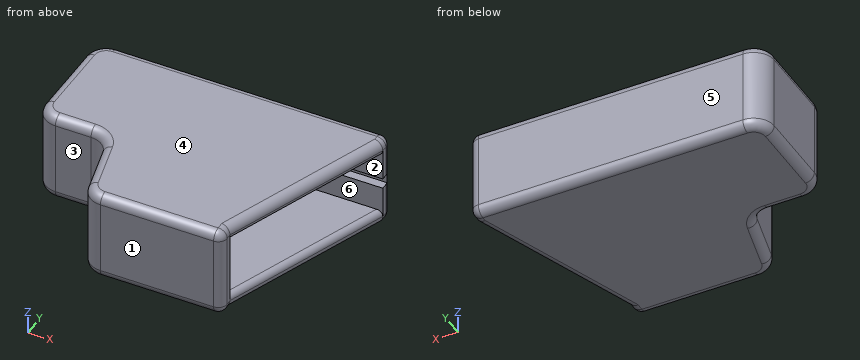
from build123d import *

# Parameters (mm, degrees)
F1_DEPTH = 21
F4_DEPTH = 5
F5_DEPTH = 5
F6_R     = 7
F7_R     = 3
F9_DEPTH = 3
F10_R    = 1.99999


# Not quite as in the source:
# - a fillet or chamfer is up to 0.001 mm smaller than in the source, because OpenCascade refuses the exact size


with BuildPart() as f1:
    # F0 (on Top) → F1 (new body)
    with BuildSketch(Plane.XY):
        Polygon((-23.5, 30), (71.5, 30), (71.5, 35), (-28.5, 35), (-28.5, -5), (-3.906596233, -5), (3.1079638678, -33.1388689644), (50.2020280941, -33.1388689644), (50.0145601007, -28.1388689644), (7.0145601007, -28.1388689644), (0, 0), (-23.5, 0), align=None)
    extrude(amount=F1_DEPTH)

    # F3 (on face) → F4 (join)
    with BuildSketch(Plane.XY.offset(21)):
        Polygon((71.5, 35), (-28.5, 35), (-28.5, -5), (-3.906596233, -5), (3.1079638678, -33.1388689644), (50.2020280941, -33.1388689644), (50.0145601007, -28.1388689644), (71.5, 30), align=None)
    extrude(amount=F4_DEPTH)

    # F2 (on face) → F5 (join)
    with BuildSketch(Plane(origin=(0, 0, 0), x_dir=(1, 0, 0), z_dir=(0, 0, -1))):
        Polygon((-28.5, -35), (71.5, -35), (71.5, -30), (50.0145601007, 28.1388689644), (50.2020280941, 33.1388689644), (3.1079638678, 33.1388689644), (-3.906596233, 5), (-28.5, 5), align=None)
    extrude(amount=F5_DEPTH)

    # F6
    f6_edges = [f1.edges().sort_by_distance(p)[0] for p in [
        (0, 0, 10.5),
        (-3.906596, -5, 10.5),
        (7.01456, -28.138869, 10.5),
        (3.107964, -33.138869, 10.5),
        (-28.5, -5, 10.5),
        (-28.5, 35, 10.5),
        (-23.5, 0, 10.5),
    ]]
    fillet(f6_edges, radius=F6_R)

    # F7
    f7_edges = [f1.edges().sort_by_distance(p)[0] for p in [
        (25, 35, 26),
        (25, 35, -5),
        (71.5, 35, 10.5),
        (-26.449747, 32.949747, 26),
        (71.5, 32.5, 26),
        (-28.5, 15, 26),
        (60.75728, 0.930566, 26),
        (-26.449747, -2.949747, 26),
        (50.108294, -30.638869, 26),
        (-15.437915, -5, 26),
        (29.389613, -33.138869, 26),
        (-5.066085, -6.484015, 26),
        (4.267453, -31.654854, 26),
        (-0.399316, -19.069434, 26),
        (-15.437915, -5, -5),
        (-5.066085, -6.484015, -5),
        (-26.449747, -2.949747, -5),
        (-0.399316, -19.069434, -5),
        (-28.5, 15, -5),
        (4.267453, -31.654854, -5),
        (-26.449747, 32.949747, -5),
        (29.389613, -33.138869, -5),
        (50.108294, -30.638869, -5),
        (71.5, 32.5, -5),
        (60.75728, 0.930566, -5),
        (50.202028, -33.138869, 10.5),
    ]]
    fillet(f7_edges, radius=F7_R)

    # F8 (on face) → F9 (cut)
    with BuildSketch(Plane.XZ.offset(-30)):
        Polygon((-23.5, 12.25), (-23.5, 10.5), (-23.5, 8.75), (74.1642639041, 8.75), (74.1642639041, 12.25), align=None)
    extrude(amount=-F9_DEPTH, mode=Mode.SUBTRACT)

    # F10 (radius 2 in the source; OpenCascade refuses exactly that, so slightly less here)
    f10_edges = [f1.edges().sort_by_distance(p)[0] for p in [
        (60.75728, 0.930566, 21),
        (60.75728, 0.930566, 0),
    ]]
    fillet(f10_edges, radius=F10_R)


solid = f1.part
Work out the finished part from the listing and answer in its coordinate system (mm). Face numbers are marked on the shaded views. A direction names the side the tool comes from. Coordinates: 2 decimals unless noted, no trailing zeros. Loops run counter-clockwise (first coordinate to the right, second up) from the corner with the lowest first, then second, coordinate; pieces in that order, holes last. Notation, with made-up numbers: (-5, -23) -> (37, -23) arc R33 ccw to (37, 7) -> close; hole circle Ø5 at (-22, 63.5). An arc over 180 degrees is marked (long way). Write each question's results on one line, items separated by ' | '. Start each with the question number.
1) Flat-ended cylindrical pins translate along their axes: P1, Ø4, axis at y = 9, z = 20.5, coming from the +X side; P2, Ø1.5, axis at y = 26.5, z = 2.5, coming from the +X side; P3, Ø3.5, axis at x = -16.5, z = 4.5, coming from the -Y side. Find the tip coordinate at first contact, or state that the pin passes through.
2) The mould has two halves that part along Y. Classify the marked faces 4, 5 and 6: pulls with the +Y half, pulls with the -Y half, needs draft (parallel to the pull), parting line crosses it, or undercut.
3) Find section A-A on x = 39.5. Determine the outline of the cut face in (y, z), then the cut area to 3 significant figures.
4) Consider line 1 along Z through (x, y) = (-10, 22.5); line 2 along Y through (x, z) = (46.5, 17); line 3 along Y through (x, z) = (-16.5, 1). Determine where each line is inside the solid, lowest interval first.
5) Find section C-C on z = -3. Determine the outline of the cut face in (x, y), then the cut area to 3 significant figures.
6) Find section B-B on z = 7. Determine the outline of the cut face in (x, y), then the cut area to 3 significant figures.
7) For the marked faces 1, 2 and 3, determine the directions among +Z, -Z, +X, -X, +Y, -Y from which every point of the face is accessible in a straight line to the end or side of a thin tool.
Response values:
1) P1: stops at x = 63.96 | P2: stops at x = -23.5 | P3: stops at y = -5
2) face 4: needs draft | face 5: pulls with the +Y half | face 6: undercut
3) outline: (-33.14, -2) arc R3 ccw to (-30.14, -5) -> (32, -5) arc R3 ccw to (35, -2) -> (35, 23) arc R3 ccw to (32, 26) -> (-30.14, 26) arc R3 ccw to (-33.14, 23) -> close; hole (-28.14, 0) -> (30, 0) -> (30, 8.75) -> (33, 8.75) -> (33, 12.25) -> (30, 12.25) -> (30, 21) -> (-28.14, 21) -> close | area: 873 mm^2
4) line 1: z = -5 to 0, 21 to 26 | line 2: y = -33.14 to -28.14, 30 to 35 | line 3: y = -5 to 0, 30 to 35
5) outline: (-28.33, 2) arc R6.83 ccw to (-21.5, -4.83) -> (-9.38, -4.83) arc R7.17 cw to (-2.42, -10.27) -> (1.95, -27.79) arc R6.83 ccw to (8.58, -32.97) -> (47.09, -32.97) arc R2.83 ccw to (49.91, -30.03) -> (49.84, -28.11) -> (71.33, 30.03) -> (71.33, 32) arc R2.83 ccw to (68.5, 34.83) -> (-21.5, 34.83) arc R6.83 ccw to (-28.33, 28) -> close | area: 5,220 mm^2
6) outline: (-28.5, 2) arc R7 ccw to (-21.5, -5) -> (-9.38, -5) arc R7 cw to (-2.58, -10.31) -> (1.79, -27.83) arc R7 ccw to (8.58, -33.14) -> (47.09, -33.14) arc R3 ccw to (50.09, -30.03) -> (50.01, -28.14) -> (12.48, -28.14) arc R7 cw to (5.69, -22.83) -> (1.32, -5.31) arc R7 ccw to (-5.47, 0) -> (-16.5, 0) arc R7 cw to (-23.5, 7) -> (-23.5, 30) -> (71.5, 30) -> (71.5, 32) arc R3 ccw to (68.5, 35) -> (-21.5, 35) arc R7 ccw to (-28.5, 28) -> close | area: 1,140 mm^2
7) face 1: +Z, -Z, +X, -X, -Y | face 2: +X | face 3: +Z, -Z, -X, -Y
